```python
from build123d import *

# Parameters (mm, degrees)
ESQUISSE1_W             = 108.59
ESQUISSE1_H             = 108.59
ESQUISSE1_R             = 1.8
BOSS_EXTRU_1_DEPTH      = 5
ESQUISSE2_W             = 54.295
ESQUISSE2_H             = 7
BOSS_EXTRU_2_DEPTH      = 35
ESQUISSE3_R             = 1
BOSS_EXTRU_3_DEPTH      = 8
ESQUISSE4_W             = 8.59995714
ESQUISSE4_H             = 23.592650329
ENL_V_MAT_EXTRU_1_DEPTH = 5
ESQUISSE8_W             = 5
ESQUISSE8_H             = 33
ENL_V_MAT_EXTRU_2_DEPTH = 54.3
ESQUISSE9_W             = 38
ESQUISSE9_H             = 30
ENL_V_MAT_EXTRU_3_DEPTH = 134.157940401
ENL_V_MAT_EXTRU_4_DEPTH = 74.3


with BuildPart() as part:
    # Esquisse1 → Boss.-Extru.1 (new body)
    with BuildSketch(Plane(origin=(0, 0, 0), x_dir=(-1, 0, 0), z_dir=(0, 0, 1))):
        with Locations((42.529454852, 77.182817805)):
            Rectangle(ESQUISSE1_W, ESQUISSE1_H)
        with Locations(Location((-1.765545148, 121.477817805, 0), (0, 0, 180))):
            Circle(ESQUISSE1_R, mode=Mode.SUBTRACT)
        with Locations(Location((86.824454852, 121.477817805, 0), (0, 0, 180))):
            Circle(ESQUISSE1_R, mode=Mode.SUBTRACT)
        with Locations(Location((86.824454852, 32.887817805, 0), (0, 0, 180))):
            Circle(ESQUISSE1_R, mode=Mode.SUBTRACT)
        with Locations(Location((-1.765545148, 32.887817805, 0), (0, 0, 180))):
            Circle(ESQUISSE1_R, mode=Mode.SUBTRACT)
        with Locations(Location((42.529454852, 32.887817805, 0), (0, 0, 180))):
            Circle(ESQUISSE1_R, mode=Mode.SUBTRACT)
        with Locations(Location((42.529454852, 121.477817805, 0), (0, 0, 180))):
            Circle(ESQUISSE1_R, mode=Mode.SUBTRACT)
    extrude(amount=BOSS_EXTRU_1_DEPTH)

    # Esquisse2 → Boss.-Extru.2 (add)
    with BuildSketch(Plane.XY.offset(5)):
        with Locations((-15.381954852, -97.182817805)):
            Rectangle(ESQUISSE2_W, ESQUISSE2_H)
        Polygon((-42.529454852, -60.682817805), (-42.529454852, -53.682817805), (-49.529454852, -53.682817805), (-49.529454852, -100.682817805), (-42.529454852, -100.682817805), (-42.529454852, -93.682817805), (-42.529454852, -77.182817805), align=None)
        with Locations((-15.381954852, -57.182817805)):
            Rectangle(ESQUISSE2_W, ESQUISSE2_H)
    extrude(amount=BOSS_EXTRU_2_DEPTH)

    # Esquisse3 → Boss.-Extru.3 (add)
    with BuildSketch(Plane.XY.offset(40)):
        Polygon((11.765545148, -53.682817805), (-49.529454852, -53.682817805), (-49.529454852, -100.682817805), (11.765545148, -100.682817805), (11.765545148, -88.982817805), (-42.529454852, -88.982817805), (-42.529454852, -65.390167476), (11.765545148, -65.390167476), align=None)
        with Locations((-24.229454852, -90.682817805)):
            Circle(ESQUISSE3_R, mode=Mode.SUBTRACT)
        with BuildLine():
            ThreePointArc((-15.229454852, -90.682817805), (-16.229454852, -91.682817805), (-17.229454852, -90.682817805))
            ThreePointArc((-17.229454852, -90.682817805), (-16.229454852, -89.682817805), (-15.229454852, -90.682817805))
        make_face(mode=Mode.SUBTRACT)
        with BuildLine():
            ThreePointArc((-7.229454852, -90.682817805), (-8.229454852, -91.682817805), (-9.229454852, -90.682817805))
            ThreePointArc((-9.229454852, -90.682817805), (-8.229454852, -89.682817805), (-7.229454852, -90.682817805))
        make_face(mode=Mode.SUBTRACT)
        with Locations((-0.229454852, -90.682817805)):
            Circle(ESQUISSE3_R, mode=Mode.SUBTRACT)
        with Locations((-24.229454852, -63.682817805)):
            Circle(ESQUISSE3_R, mode=Mode.SUBTRACT)
        with BuildLine():
            ThreePointArc((-15.229454852, -63.682817805), (-16.229454852, -64.682817805), (-17.229454852, -63.682817805))
            ThreePointArc((-17.229454852, -63.682817805), (-16.229454852, -62.682817805), (-15.229454852, -63.682817805))
        make_face(mode=Mode.SUBTRACT)
        with BuildLine():
            ThreePointArc((-7.229454852, -63.682817805), (-8.229454852, -64.682817805), (-9.229454852, -63.682817805))
            ThreePointArc((-9.229454852, -63.682817805), (-8.229454852, -62.682817805), (-7.229454852, -63.682817805))
        make_face(mode=Mode.SUBTRACT)
        with Locations((-0.229454852, -63.682817805)):
            Circle(ESQUISSE3_R, mode=Mode.SUBTRACT)
    extrude(amount=BOSS_EXTRU_3_DEPTH)

    # Esquisse4 → Enl_v. mat.-Extru.1 (cut)
    with BuildSketch(Plane.XY.offset(5)):
        with Locations((-18.074099951, -77.186492641)):
            Rectangle(ESQUISSE4_W, ESQUISSE4_H)
    extrude(amount=-ENL_V_MAT_EXTRU_1_DEPTH, mode=Mode.SUBTRACT)

    # Esquisse5 → Lissage3 section 0
    with BuildSketch(Plane.ZY.offset(49.529454852)):
        with BuildLine():
            Line((48, -100.682817805), (38, -100.682817805))
            Line((38, -100.682817805), (38, -53.682817805))
            Line((38, -53.682817805), (48, -53.682817805))
            Line((48, -53.682817805), (48, -100.682817805))
        make_face()
    # Esquisse6 → Lissage3 section 1
    with BuildSketch(Plane.XY.offset(5)):
        with BuildLine():
            Line((-74.529454852, -115.182817805), (-74.529454852, -39.182817805))
            Line((-74.529454852, -39.182817805), (-70.204298905, -41.691408254))
            Line((-70.204298905, -41.691408254), (-70.204298905, -112.674227356))
            Line((-70.204298905, -112.674227356), (-74.529454852, -115.182817805))
        make_face()
    loft()

    # Esquisse8 → Enl_v. mat.-Extru.2 (cut)
    with BuildSketch(Plane(origin=(11.765545148, 0, 0), x_dir=(0, 0, -1), z_dir=(1, 0, 0))):
        with Locations((-42.5, -77.182817805)):
            Rectangle(ESQUISSE8_W, ESQUISSE8_H)
    extrude(amount=-ENL_V_MAT_EXTRU_2_DEPTH, mode=Mode.SUBTRACT)

    # Esquisse9 → Enl_v. mat.-Extru.3 (cut, through all)
    with BuildSketch(Plane(origin=(0, -53.682817805, 0), x_dir=(1, 0, 0), z_dir=(0, 1, 0))):
        with Locations((-12.943096448, -30)):
            Rectangle(ESQUISSE9_W, ESQUISSE9_H)
    extrude(amount=-ENL_V_MAT_EXTRU_3_DEPTH, mode=Mode.SUBTRACT)

    # Esquisse10 → Enl_v. mat.-Extru.4 (cut)
    with BuildSketch(Plane.XY.offset(5)):
        Polygon((-13.774121381, -65.390167476), (11.765545148, -65.390167476), (11.765545148, -70.390167476), (-5.389368853, -70.390167476), (-13.774121381, -75.390167476), align=None)
    extrude(amount=-ENL_V_MAT_EXTRU_4_DEPTH, mode=Mode.SUBTRACT)


solid = part.part
```
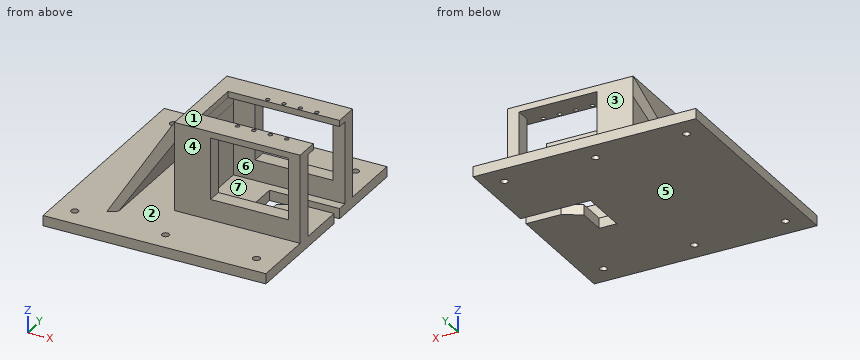
Could you check a few things on this model? Use its own coordinates, in mm. Face numbers are marked on the shaded views. A direction names the side the tool comes from. Give positions to 0.01 mm unless a question says otherwise; leave off trailing zeros. Order: outer loops, then holes, each group sorted by start corner. A loop starts at its lowest first (then second) coordinate and runs counter-clockwise, first axis right, second up.
Q1. Suppose I cut it at A-A, the plane x = -34. Write out the boundary of the cut face in (y, z).
Q2. If I drill on line 1 along Z through (x, y) = (-11.5, -54); line 2 along Y through (x, z) = (-28, 14); line 3 along X through (y, z) = (-97, 23.5), over which ranges is the centre line in solid material (lowest first)?
Q3. Suppose I cut it at D-D, the plane y = -37. Write out the boundary of the cut face in (x, z).
Q4. I'm going to push flat-ended pins straight in: P1, Ø1.2, axis at x = -24.23, y = -90.68, coming from the +Z side; P2, Ø4, axis at y = -70, z = 41.5, coming from the +X side; P3, Ø10, axis at y = -56, z = 23.5, coming from the -X side. Where does each tip first touch, or does it pass through?
Q5. For the marked faces 1, 2 and 3, which set-ups out of +Z, -Z, +X, -X, +Y, -Y let a thin tool reach every point of the face, with its end or its side?
Q6. Suppose I cut it at B-B, the plane y = -98.5. Count the separate pieces of the cut face and the enclosed holes in it, and give its area (4 significant figures).
Q7. We'd pull the mould along Y, two halves only. Please class the marked faces 4, 5, 6 and 7: +Y half, -Y half, draft (parallel to the pull), parting line (faces both ways), or undercut.
Solution:
1. outline: (-131.48, 0) - (-22.89, 0) - (-22.89, 5) - (-53.68, 5) - (-53.68, 48) - (-65.39, 48) - (-65.39, 45) - (-60.68, 45) - (-60.68, 5) - (-93.68, 5) - (-93.68, 45) - (-88.98, 45) - (-88.98, 48) - (-100.68, 48) - (-100.68, 5) - (-131.48, 5) - close
2. line 1: z = 0 to 15, 45 to 48
2. line 2: y = -100.68 to -93.68, -60.68 to -53.68
2. line 3: x = -63.77 to -58.61, -49.53 to -31.94, 6.06 to 11.77
3. outline: (-96.82, 0) - (11.77, 0) - (11.77, 5) - (-96.82, 5) - close
4. P1: stops at z = 5
4. P2: stops at x = -42.53
4. P3: stops at x = -66.68
5. face 1: +Z, +X, -X, +Y, -Y
5. face 2: none
5. face 3: +Z, +X, +Y
6. separate pieces: 1
6. enclosed holes: 2
6. area: 2,235 mm2
7. face 4: -Y half
7. face 5: draft
7. face 6: undercut
7. face 7: undercut
